Geometry check sheet. Reference: the model listing, model coordinates, mm. Give positions to 0.01 mm unless a question says otherwise; leave off trailing zeros. Order: outer loops, then holes, each group sorted by start corner. A loop starts at its lowest first (then second) coordinate and runs counter-clockwise, first axis right, second up.
from build123d import *

# Parameters (mm, degrees)
SKETCH1_R           = 12.5
BOSS_EXTRUDE1_DEPTH = 600
SKETCH5_R           = 5
CUT_EXTRUDE2_DEPTH  = 685
CHAMFER1_SIZE       = 2
CHAMFER1_SIZE2      = 1.154700538


with BuildPart() as part:
    # Sketch1 → Boss-Extrude1 (new body)
    with BuildSketch(Plane(origin=(0, 0, 0), x_dir=(1, 0, 0), z_dir=(0, 1, 0))):
        with Locations(Location((0, 0, 0), (0, 0, 270))):
            Circle(SKETCH1_R)
    extrude(amount=BOSS_EXTRUDE1_DEPTH)

    # Sketch5 → Cut-Extrude2 (cut)
    with BuildSketch(Plane(origin=(8.266546367, 600, 9.376257844), x_dir=(0.7501006275419531, 0, -0.6613237093596208), z_dir=(0.6613237093596208, 0, 0.7501006275419531))):
        with Locations((0, -15)):
            Circle(SKETCH5_R)
    extrude(amount=-CUT_EXTRUDE2_DEPTH, mode=Mode.SUBTRACT)

    # Chamfer1
    chamfer1_edges = [part.edges().sort_by_distance(p)[0] for p in [
        (0, 0, -12.5),
    ]]
    chamfer1_side = [part.faces().sort_by_distance(p)[0] for p in [
        (0, 0, 0),
    ]]
    chamfer(chamfer1_edges, length=CHAMFER1_SIZE, length2=CHAMFER1_SIZE2, reference=chamfer1_side[0])


solid = part.part
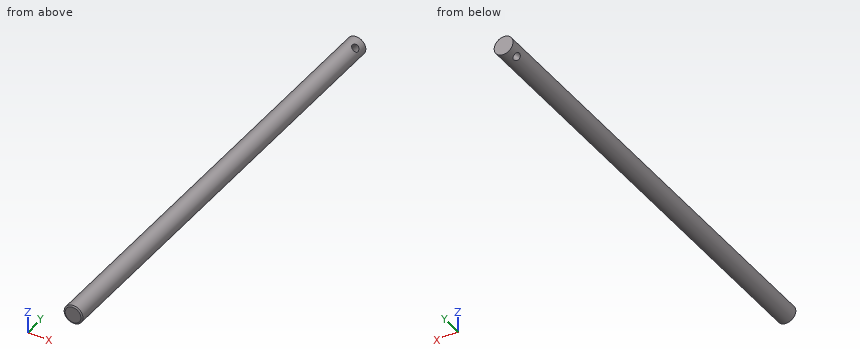
Item 1: Sectioned sample at A-A (y = 420). Enter the section's corners in (x, z).
Reported:
outline: circle Ø25 at (0, 0)
Item 2: Scan lines: L1, parallel to X at y = 141, z = 3.5; L2, parallel to Y at x = -2.5, z = -0.5; L3, parallel to Y at x = -1.5, z = -2.25. Record each from-to range of solid material in increasing order.
Reported:
L1: x = -12 to 12
L2: y = 0 to 580.24, 589.76 to 600
L3: y = 0 to 580.01, 589.99 to 600
Item 3: Gauge pin test, flat ends, axial feed: pin 1 (12 mm diameter, centred on x = -6, y = 242.5, fed in from -Z); pin 2 (10 mm diameter, centred on y = 171.5, z = -7.5, fed in from +X); pin 3 (1 mm diameter, centred on y = 365.5, z = 9.5, fed in from +X). Record the tip position at first contact, or that the pin passes through.
Reported:
pin 1: stops at z = -12.5
pin 2: stops at x = 12.25
pin 3: stops at x = 8.67
